from build123d import *

# Parameters (mm, degrees)
BOSS_EXTRUDE1_DEPTH = 127
FILLET2_R           = 63.5


with BuildPart() as part:
    # Sketch1 → Boss-Extrude1 (new body)
    with BuildSketch(Plane.XY):
        Polygon((-84.386835568, -262.623028831), (-84.386835568, -173.723028831), (-401.886835568, -173.723028831), (-401.886835568, -1172.197028831), (461.713164432, -1172.197028831), (461.713164432, -173.723028831), (144.213164432, -173.723028831), (144.213164432, -262.623028831), (372.813164432, -262.623028831), (372.813164432, -1083.297028831), (-312.986835568, -1083.297028831), (-312.986835568, -262.623028831), align=None)
    extrude(amount=BOSS_EXTRUDE1_DEPTH)

    # Fillet2
    fillet2_edges = [part.edges().sort_by_distance(p)[0] for p in [
        (302.963164432, -173.723028831, 0),
        (302.963164432, -173.723028831, 127),
        (-243.136835568, -173.723028831, 0),
        (-243.136835568, -173.723028831, 127),
        (-401.886835568, -672.960028831, 127),
        (-401.886835568, -672.960028831, 0),
        (461.713164432, -672.960028831, 127),
        (461.713164432, -672.960028831, 0),
        (29.913164432, -1172.197028831, 0),
        (29.913164432, -1172.197028831, 127),
    ]]
    fillet(fillet2_edges, radius=FILLET2_R - 0.0001)  # a hair under: the kernel refuses the full size


solid = part.part
Here's how the part is built. I have some questions about the finished solid (model axes, mm). A direction names the side the tool comes from. Round coordinates to 2 decimals unless told otherwise and drop trailing zeros. Order: outer loops, then holes, each group sorted by start corner. A loop starts at its lowest first (then second) coordinate and runs counter-clockwise, first axis right, second up. Notation, with made-up numbers: (42.25, 41.5) -> (69.25, 41.5) arc R9 cw to (69.25, 47.5) -> close; hole circle Ø4 at (29.25, 36.25). An arc over 180 degrees is marked (long way). Use CSV: the item, a comma, the result in double quotes.
1. Thinking about a two-plate mould opening in X: for faces 1 (the face through (-383.779, -679.949, 19.095)), 2 (the face through (372.813, -667, 63)), 3 (the face through (-245.359, -191.831, 19.095)), which applies, pulls with the +X half, pulls with the -X half, needs draft (parallel to the pull), parting line crosses it, or undercut?
Recorded:
face 1,"pulls with the -X half"
face 2,"undercut"
face 3,"needs draft"
2. I want a section at C-C on z = 48. List the corners of the cut face in (x, y) for me, and give its area (3 significant figures).
Recorded:
outline,"(-399.97, -1170.28) -> (459.79, -1170.28) -> (459.79, -175.64) -> (144.21, -175.64) -> (144.21, -262.62) -> (372.81, -262.62) -> (372.81, -1083.3) -> (-312.99, -1083.3) -> (-312.99, -262.62) -> (-84.39, -262.62) -> (-84.39, -175.64) -> (-399.97, -175.64) -> close"
area,"272,000 mm2"
3. I need wall thicknesses on line 1 along X through (y, z) = (-864, 63.5); line 2 along X through (y, z) = (-295, 59); line 3 along Y through (x, z) = (-272.5, 96). Which ranges of each line are inside material? Lowest first, please.
Recorded:
line 1,"x = -401.89 to -312.99, 372.81 to 461.71"
line 2,"x = -401.73 to -312.99, 372.81 to 461.55"
line 3,"y = -1163.25 to -1083.3, -262.62 to -182.67"
4. Which directions (+Z, -Z, +X, -X, +Y, -Y) give clear straight access to the entire face, cutting with the end or side of a thin tool? Please do faces 4 (the face through (300.741, -191.831, 107.905)), 5 (the face through (-84.387, -229, 63)), 6 (the face through (257, -262.623, 63)).
Recorded:
face 4,"+Z, +X, -X, +Y"
face 5,"+Z, -Z, +Y"
face 6,"+Z, -Z"
5. I'm going to push flat-ended pins straight in: P1, Ø4, axis at y = -519.5, z = 68.5, coming from the -X side; P2, Ø12, axis at x = 223.5, z = 41, coming from the -Y side; P3, Ø6, axis at x = 220.5, z = 52.5, coming from the -Y side. Where does each tip first touch, or does it pass through?
Recorded:
P1,"stops at x = -401.82"
P2,"stops at y = -1170.02"
P3,"stops at y = -1171.69"
